Part model, mm, in its own coordinate system. A direction names the side the tool comes from. Coordinates: 2 decimals unless noted, no trailing zeros. Loops run counter-clockwise (first coordinate to the right, second up) from the corner with the lowest first, then second, coordinate; pieces in that order, holes last. Notation, with made-up numbers: (-33, 9) -> (-5, 9) arc R7 ccw to (-5, 21) -> close; hole circle Ø4 at (16.25, -6). An arc over 180 degrees is marked (long way). One line per item, written item: value. Start each with the question number.
from build123d import *

# Parameters (mm, degrees)
SKETCH2_W                    = 75
SKETCH2_H                    = 130
BASE_FLANGE1_DEPTH           = 0.6
TAB2_START                   = -0.6
TAB2_OUTLINE_W               = 76.2
TAB2_OUTLINE_H               = 15
TAB2_DEPTH                   = 0.6
CUT_EXTRUDE1_REACH           = 201.404
SKETCH10_R                   = 2.5
EDGE_FLANGE1_STRIP_W         = 3.8732
EDGE_FLANGE1_STRIP_H         = 0.6
EDGE_FLANGE1_STRIP_CUT_DEPTH = 151.2
EDGE_FLANGE1_DEPTH           = 151.2
EDGE_FLANGE2_DEPTH           = 72.2634


# Read off the part's stored shape, not the designer's step: Tab2
# Sheet-metal steps are written as plain solids
with BuildPart() as part:
    # Sketch2 → Base-Flange1 (new body)
    with BuildSketch(Plane.XY):
        with Locations((37.5, 65)):
            Rectangle(SKETCH2_W, SKETCH2_H)
    extrude(amount=-BASE_FLANGE1_DEPTH)

    # Tab2 outline → Tab2 (add)
    with BuildSketch(Plane.XY.offset(TAB2_START)):
        with Locations((113.1, 7.5)):
            Rectangle(TAB2_OUTLINE_W, TAB2_OUTLINE_H)
    extrude(amount=TAB2_DEPTH)

    # Sketch10 → Cut-Extrude1 (cut, up to next)
    with BuildSketch(Plane(origin=(0, 0, -0.6), x_dir=(-1, 0, 0), z_dir=(0, 0, -1)), mode=Mode.PRIVATE) as cut_extrude1_sk1:
        with Locations((-22.5, 65)):
            Circle(SKETCH10_R)
    cut_extrude1_tool1 = extrude(cut_extrude1_sk1.sketch, amount=-CUT_EXTRUDE1_REACH, mode=Mode.PRIVATE) & part.part
    # Sketch10 → Cut-Extrude1 (cut, up to next)
    with BuildSketch(Plane(origin=(0, 0, -0.6), x_dir=(-1, 0, 0), z_dir=(0, 0, -1)), mode=Mode.PRIVATE) as cut_extrude1_sk2:
        with Locations((-52.5, 115)):
            Circle(SKETCH10_R)
    cut_extrude1_tool2 = extrude(cut_extrude1_sk2.sketch, amount=-CUT_EXTRUDE1_REACH, mode=Mode.PRIVATE) & part.part
    # Sketch10 → Cut-Extrude1 (cut, up to next)
    with BuildSketch(Plane(origin=(0, 0, -0.6), x_dir=(-1, 0, 0), z_dir=(0, 0, -1)), mode=Mode.PRIVATE) as cut_extrude1_sk3:
        with Locations((-52.5, 65)):
            Circle(SKETCH10_R)
    cut_extrude1_tool3 = extrude(cut_extrude1_sk3.sketch, amount=-CUT_EXTRUDE1_REACH, mode=Mode.PRIVATE) & part.part
    # Sketch10 → Cut-Extrude1 (cut, up to next)
    with BuildSketch(Plane(origin=(0, 0, -0.6), x_dir=(-1, 0, 0), z_dir=(0, 0, -1)), mode=Mode.PRIVATE) as cut_extrude1_sk4:
        with Locations((-22.5, 115)):
            Circle(SKETCH10_R)
    cut_extrude1_tool4 = extrude(cut_extrude1_sk4.sketch, amount=-CUT_EXTRUDE1_REACH, mode=Mode.PRIVATE) & part.part
    add(cut_extrude1_tool1.solids().sort_by_distance((22.5, 65, -0.6))[0], mode=Mode.SUBTRACT)
    add(cut_extrude1_tool2.solids().sort_by_distance((52.5, 115, -0.6))[0], mode=Mode.SUBTRACT)
    add(cut_extrude1_tool3.solids().sort_by_distance((52.5, 65, -0.6))[0], mode=Mode.SUBTRACT)
    add(cut_extrude1_tool4.solids().sort_by_distance((22.5, 115, -0.6))[0], mode=Mode.SUBTRACT)

    # Edge-Flange1 strip (across the edge) → Edge-Flange1 strip cut (cut)
    with BuildSketch(Plane.YZ):
        with Locations((-0.6, -0.3)):
            Rectangle(EDGE_FLANGE1_STRIP_W, EDGE_FLANGE1_STRIP_H)
    extrude(amount=EDGE_FLANGE1_STRIP_CUT_DEPTH, mode=Mode.SUBTRACT)

    # Edge-Flange1 section (across the edge) → Edge-Flange1 (add)
    with BuildSketch(Plane.YZ):
        with BuildLine():
            Line((0, 0.7366), (0, 73))
            Line((0, 73), (0.6, 73))
            Line((0.6, 73), (0.6, 0.7366))
            ThreePointArc((0.6, 0.7366), (0.815745145, 0.215745145), (1.3366, 0))
            Line((1.3366, 0), (1.3366, -0.6))
            ThreePointArc((1.3366, -0.6), (0.391481076, -0.208518924), (0, 0.7366))
        make_face()
    extrude(amount=EDGE_FLANGE1_DEPTH)

    # Edge-Flange2 section (across the edge) → Edge-Flange2 (add)
    with BuildSketch(Plane(origin=(-0.7366, 0.6, 0.7366), x_dir=(1, 0, 0), z_dir=(0, 0, 1))):
        with BuildLine():
            Line((-0.6, 0.7366), (-0.6, 9.4))
            Line((-0.6, 9.4), (0, 9.4))
            Line((0, 9.4), (0, 0.7366))
            ThreePointArc((0, 0.7366), (0.215745145, 0.215745145), (0.7366, 0))
            Line((0.7366, 0), (0.7366, -0.6))
            ThreePointArc((0.7366, -0.6), (-0.208518924, -0.208518924), (-0.6, 0.7366))
        make_face()
    extrude(amount=EDGE_FLANGE2_DEPTH)


solid = part.part
1) Tool access for faces 4 (the flat face through (75, 0.6, 37)), 5 (the flat face through (-0.737, 6, 36)), 6 (the flat face through (-1.337, 6, 36)): list every direction of +Z, -Z, +X, -X, +Y, -Y with a clear straight run to the whole face (end or side of a thin tool).
2) Pin check, flat tips, straight feed: pin 1 Ø6 at (x, y) = (22.5, 115) entering from +Z; pin 2 Ø10 at (x, z) = (86, 28) entering from +Y; pin 3 Ø0.7 at (x, z) = (121.5, -0.5) entering from +Y. Stop position of each tip, or through.
3) Slice it at B-B (y = 65). Give the cut face in (x, z), then the cut area to 3 significant figures.
4) Slice it at D-D (x = 87.5). Give the cut face in (y, z), then the cut area to 3 significant figures.
5) Pull direction Y, two halves, no side cores. Call faces 1 (the flat face through (75, 0, 36)), 2 (the cylindrical face through (52.83, 117.48, -0.3)), 3 (the flat face through (41, 67, 0)): +Y half, -Y half, draft (parallel to the pull), parting line (faces both ways), or undercut.
6) Slice it at A-A (x = 52.5). Give the cut face in (y, z).
7) Slice it at C-C (z = 55). Give the cut face in (x, y), then the cut area to 3 significant figures.
8) Probe line 1 (Y direction, x = 22.5, z = -0.35); line 2 (Y direction, x = 22.5, z = -0.3); line 3 (Y direction, x = 24, z = 31). List the from-to ranges inside material, lowest first. Write a range as from..to.
Check sheet entries:
1. face 4: +Z, +X, +Y
1. face 5: +Z, -Z, +X, +Y
1. face 6: +Z, -Z, -X, +Y, -Y
2. pin 1: stops at z = 0
2. pin 2: stops at y = 0.6
2. pin 3: stops at y = 15
3. outline: (0, -0.6) -> (20, -0.6) -> (20, 0) -> (0, 0) -> close; (25, -0.6) -> (50, -0.6) -> (50, 0) -> (25, 0) -> close; (55, -0.6) -> (75, -0.6) -> (75, 0) -> (55, 0) -> close
3. area: 39.0 mm^2
4. outline: (0, 0.74) arc R1.34 ccw to (1.34, -0.6) -> (15, -0.6) -> (15, 0) -> (1.34, 0) arc R0.74 cw to (0.6, 0.74) -> (0.6, 73) -> (0, 73) -> close
4. area: 52.5 mm^2
5. face 1: -Y half
5. face 2: undercut
5. face 3: draft
6. outline: (0, 0.74) arc R1.34 ccw to (1.34, -0.6) -> (62.5, -0.6) -> (62.5, 0) -> (1.34, 0) arc R0.74 cw to (0.6, 0.74) -> (0.6, 73) -> (0, 73) -> close; (67.5, -0.6) -> (112.5, -0.6) -> (112.5, 0) -> (67.5, 0) -> close; (117.5, -0.6) -> (130, -0.6) -> (130, 0) -> (117.5, 0) -> close
7. outline: (-1.34, 1.34) arc R1.34 ccw to (0, 0) -> (151.2, 0) -> (151.2, 0.6) -> (0, 0.6) arc R0.74 cw to (-0.74, 1.34) -> (-0.74, 10) -> (-1.34, 10) -> close
7. area: 96.9 mm^2
8. line 1: y = 0.56..62.5, 67.5..112.5, 117.5..130
8. line 2: y = 0.49..62.5, 67.5..112.5, 117.5..130
8. line 3: y = 0..0.6
